from build123d import *

# Parameters (mm, degrees)
F1_DEPTH       = 3.175
F2_D           = 2.54
F2_CSINK_D     = 9.525
F2_CSINK_ANGLE = 90
F3_D           = 7.62
F3_CSINK_D     = 9.525
F3_CSINK_ANGLE = 90


with BuildPart() as f1:
    # F0 (on Top) → F1 (new body)
    with BuildSketch(Plane.XY):
        with BuildLine():
            Line((31.75, -10.31875), (31.75, 10.31875))
            Line((31.75, 10.31875), (-31.75, 10.31875))
            Line((-31.75, 10.31875), (-31.75, -18.25625))
            ThreePointArc((-31.75, -18.25625), (-25.4, -24.60625), (-19.05, -18.25625))
            Line((-19.05, -18.25625), (-19.05, -10.31875))
            Line((-19.05, -10.31875), (31.75, -10.31875))
        make_face()
    extrude(amount=F1_DEPTH)

    # F2 (through all)
    with Locations(Plane(origin=(0, 0, 0), x_dir=(1, 0, 0), z_dir=(0, 0, -1))):
        with Locations((25.4, 3.96875), (0, -3.96875), (-25.4, 4.7241849825)):
            CounterSinkHole(F2_D / 2, F2_CSINK_D / 2, counter_sink_angle=F2_CSINK_ANGLE)

    # F3 (through all)
    with Locations(Plane(origin=(0, 0, 0), x_dir=(1, 0, 0), z_dir=(0, 0, -1))):
        with Locations((-25.4, 18.25625)):
            CounterSinkHole(F3_D / 2, F3_CSINK_D / 2, counter_sink_angle=F3_CSINK_ANGLE)


solid = f1.part
Geometry check sheet. Reference: the model listing, model coordinates, mm. A direction names the side the tool comes from. Give positions to 0.01 mm unless a question says otherwise; leave off trailing zeros. Loops run counter-clockwise (first coordinate to the right, second up) from the corner with the lowest first, then second, coordinate; pieces in that order, holes last. Notation, with made-up numbers: M 27.5,31 L 48.5,31 A23 ccw 48.5,57 Z; hole C 52,56.5 d5. An arc over 180 degrees is marked long. Answer as a JSON object with one key per item and string values. Group by question number.
Item 1: Sectioned sample at A-A on x = -25.4. Record the boundary of the cut face in (y, z) (1 decimal).
Item 2: Mould release check, pull along Y, two halves, no side actions. Record for faces 1 (the flat face through (6, -10.319, 2)), 2 (the flat face through (0, 10.319, 2)), 3 (the conical face through (23.79, -3.3, 3.02)), 4 (the flat face through (-31.75, -4, 2)): pulls with the +Y half, pulls with the -Y half, needs draft (parallel to the pull), parting line crosses it, or undercut.
Item 3: Access from +Z, -Z, +X, -X, +Y, -Y to the whole of each face (thin tool, end or side, straight path). Record for faces 5 (the cylindrical face through (-29.034, -19.401, 2.079)), 6 (the flat face through (-19.05, -14, 2)).
Item 4: Sectioned sample at C-C on x = 0. Record the boundary of the cut face in (y, z) (3 decimals), plus the area to 3 significant figures.
Item 5: Gauge pin test, flat end, axial feed: pin 1 (1.6 mm diameter, centred on y = -12.5, z = 1.5, fed in from +X). Record the tip position at first contact, or that the pin passes through.
Item 6: Sectioned sample at B-B on z = 2.65. Give the number of separate pieces and of enclosed holes in the cut face, plus the area to 3 significant figures.
Item 7: Material ranges on L1, parallel to X at y = -5, z = 0.4; L2, parallel to Y at x = -25.4, z = 2.75; L3, parallel to Y at x = 4, z = 1.7, recorded low to high.
Findings below:
{
 "1": {"outline": "M -24.6,0 L -23,0 L -22.1,1 L -22.1,3.2 L -24.6,3.2 Z; M -14.4,1 L -13.5,0 L -9.5,0 L -6.3,3.2 L -14.4,3.2 Z; M -3.1,3.2 L 0,0 L 10.3,0 L 10.3,3.2 Z"},
 "2": {"face 1": "pulls with the -Y half", "face 2": "pulls with the +Y half", "face 3": "undercut", "face 4": "needs draft"},
 "3": {"face 5": "+Z, -Z", "face 6": "+Z, -Z, +X, -Y"},
 "4": {"outline": "M -10.319,0 L -0.794,0 L 2.381,3.175 L -10.319,3.175 Z; M 5.556,3.175 L 8.731,0 L 10.319,0 L 10.319,3.175 Z", "area": "45.4 mm2"},
 "5": {"pin 1": "x = -19.05"},
 "6": {"separate pieces": "1", "enclosed holes": "4", "area": "1,390 mm2"},
 "7": {"L1": "-31.75 to -29.75, -21.05 to 21.16, 29.64 to 31.75", "L2": "-24.61 to -22.07, -14.45 to -6.74, -2.71 to 10.32", "L3": "-10.32 to 10.32"}
}
